Geometry: final body of the model. Coordinates: model frame, mm. Face numbers are marked on the shaded views. A direction names the side the tool comes from. Coordinates: 2 decimals unless noted, no trailing zeros. Write each loop counter-clockwise with the first axis right and the second up, starting at its lowest first coordinate (ties: lowest second). Pieces come first, ordered by that corner, then holes. Notation, with made-up numbers: (39.5, -31) -> (62.5, -31) arc R27 cw to (62.5, 3) -> close; hole circle Ø5 at (-13.5, -6.5). An arc over 180 degrees is marked (long way). One line per item, written item: value. Start each with the question number.
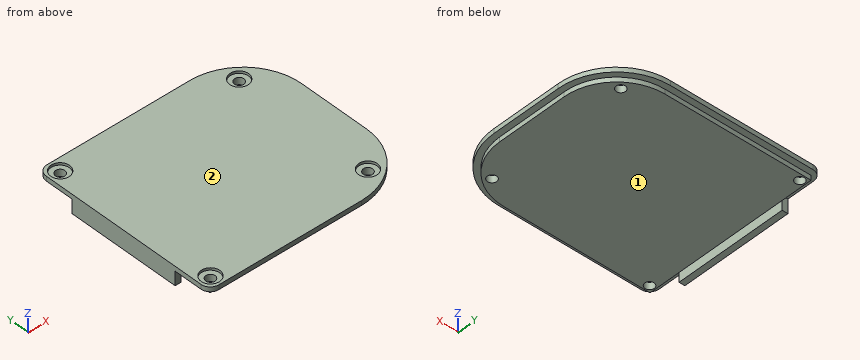
from build123d import *

# Parameters (mm, degrees)
SKETCH004_R     = 2
PAD003_DEPTH    = 2
PAD004_DEPTH    = 2
SKETCH006_W     = 2.5
SKETCH006_H     = 48
PAD005_DEPTH    = 6
SKETCH007_R     = 2
POCKET001_DEPTH = 8.001
SKETCH008_R     = 4
POCKET002_DEPTH = 1
FILLET001_R     = 4


with BuildPart() as part:
    # Sketch004 → Pad003 (new body)
    with BuildSketch(Plane.XY.offset(53)):
        with BuildLine():
            Line((20, 40), (-45, 40))
            Line((-45, 40), (-45, -40))
            Line((-45, -40), (20, -40))
            ThreePointArc((20, -40), (37.67767, -32.67767), (45, -15))
            Line((45, -15), (45, 15))
            ThreePointArc((45, 15), (37.67767, 32.67767), (20, 40))
        make_face()
        with Locations((-40, 35)):
            Circle(SKETCH004_R, mode=Mode.SUBTRACT)
        with Locations((32, 30)):
            Circle(SKETCH004_R, mode=Mode.SUBTRACT)
        with Locations((-40, -35)):
            Circle(SKETCH004_R, mode=Mode.SUBTRACT)
        with Locations((32, -30)):
            Circle(SKETCH004_R, mode=Mode.SUBTRACT)
    extrude(amount=PAD003_DEPTH)

    # Sketch005 (on Face7 of Pad003) → Pad004 (join)
    with BuildSketch(Plane(origin=(0, 0, 53), x_dir=(1, 0, 0), z_dir=(0, 0, -1))):
        with BuildLine():
            Line((-42.5, 37.5), (-42.5, -37.5))
            Line((-42.5, -37.5), (20, -37.5))
            ThreePointArc((20, -37.5), (35.909903, -30.909903), (42.5, -15))
            Line((42.5, 15), (42.5, -15))
            ThreePointArc((42.5, 15), (35.909903, 30.909903), (20, 37.5))
            Line((-42.5, 37.5), (20, 37.5))
        make_face()
    extrude(amount=PAD004_DEPTH)

    # Sketch006 (on Face4 of Pad004) → Pad005 (join)
    with BuildSketch(Plane(origin=(0, 0, 53), x_dir=(1, 0, 0), z_dir=(0, 0, -1))):
        with Locations((-43.75, 0)):
            Rectangle(SKETCH006_W, SKETCH006_H)
    extrude(amount=PAD005_DEPTH)

    # Sketch007 (on Face5 of Pad005) → Pocket001 (cut, through all)
    with BuildSketch(Plane.XY.offset(55)):
        with Locations((-40, 35)):
            Circle(SKETCH007_R)
        with Locations((-40, -35)):
            Circle(SKETCH007_R)
        with Locations((32, -30)):
            Circle(SKETCH007_R)
        with Locations((32, 30)):
            Circle(SKETCH007_R)
    extrude(amount=-POCKET001_DEPTH, mode=Mode.SUBTRACT)

    # Sketch008 (on Face5 of Pocket001) → Pocket002 (cut)
    with BuildSketch(Plane.XY.offset(55)):
        with Locations((32, 30)):
            Circle(SKETCH008_R)
        with Locations((-40, 35)):
            Circle(SKETCH008_R)
        with Locations((32, -30)):
            Circle(SKETCH008_R)
        with Locations((-40, -35)):
            Circle(SKETCH008_R)
    extrude(amount=-POCKET002_DEPTH, mode=Mode.SUBTRACT)

    # Fillet001
    fillet001_edges = [part.edges().sort_by_distance(p)[0] for p in [
        (-45, 40, 54),
        (-45, -40, 54),
    ]]
    fillet(fillet001_edges, radius=FILLET001_R)


solid = part.part
Q1. Cut plane B-B on y = 8. Output: boundary loops of the cut face in (x, z), and give its area (3 significant figures).
Q2. Cut plane D-D on x = 4.5. Output: boundary loops of the cut face in (y, z).
Q3. Cut plane A-A on x = -40. Output: boundary loops of the cut face in (y, z).
Q4. Access query for the marked faces 1 and 2. Directions: +Z, -Z, +X, -X, +Y, -Y. A direction counts if a zero-diameter tool reaches every point of the face in a straight line with its end or side. Return the directions, or none.
Q5. Cut plane C-C on y = -30. Output: boundary loops of the cut face in (x, z).
Q6. First-contact query: P1, Ø0.6, axis at y = 1.5, z = 52, coming from the +X side; P2, Ø1.5, axis at x = 22, y = -18, coming from the -Z side; P3, Ø1.6, axis at y = -30.5, z = 52, coming from the -X side; P4, Ø3, axis at x = -40, y = -35, coming from the -Z side. Flat tips, straight axial feed; report the tip coordinate or a pass-through.
Q7. Line query: L1, parallel to Y at x = -40, z = 53.3; L2, parallel to Y at x = -40, z = 52.05; L3, parallel to Z at x = 24, y = 0.5. Output: solid intervals per line, ascending. Write a range as from..to.
Solution:
1. outline: (-45, 47) -> (-42.5, 47) -> (-42.5, 51) -> (42.5, 51) -> (42.5, 53) -> (45, 53) -> (45, 55) -> (-45, 55) -> close
1. area: 365 mm²
2. outline: (-40, 53) -> (-37.5, 53) -> (-37.5, 51) -> (37.5, 51) -> (37.5, 53) -> (40, 53) -> (40, 55) -> (-40, 55) -> close
3. outline: (-40, 53) -> (-37.5, 53) -> (-37.5, 51) -> (-37, 51) -> (-37, 54) -> (-39, 54) -> (-39, 55) -> (-40, 55) -> close; (-33, 51) -> (33, 51) -> (33, 54) -> (31, 54) -> (31, 55) -> (-31, 55) -> (-31, 54) -> (-33, 54) -> close; (37, 51) -> (37.5, 51) -> (37.5, 53) -> (40, 53) -> (40, 55) -> (39, 55) -> (39, 54) -> (37, 54) -> close
4. face 1: -Z, +X, +Y, -Y
4. face 2: +Z, +X, -X, +Y, -Y
5. outline: (-45, 53) -> (-42.5, 53) -> (-42.5, 51) -> (30, 51) -> (30, 54) -> (28, 54) -> (28, 55) -> (-45, 55) -> close; (34, 51) -> (36.77, 51) -> (36.77, 53) -> (40, 53) -> (40, 55) -> (36, 55) -> (36, 54) -> (34, 54) -> close
6. P1: x = 42.5
6. P2: z = 51
6. P3: x = -42.5
6. P4: through
7. L1: -40..-37, -33..33, 37..40
7. L2: -37.5..-37, -33..33, 37..37.5
7. L3: 51..55
